Input: part model. Units: mm. Frame: model coordinates. A direction names the side the tool comes from. Give positions to 0.01 mm unless a question says otherwise; leave off trailing zeros. Use CSV: the item, a comma, the result in double quotes.
```python
from build123d import *

# Parameters (mm, degrees)
F0_R     = 3.1
F0_R_2   = 1.75
F1_DEPTH = 16.8
F3_DEPTH = 4
F4_R     = 4
F5_DEPTH = 25
F6_R     = 3


with BuildPart() as f1:
    # F0 (on Top) → F1 (new body)
    with BuildSketch(Plane.XY):
        with BuildLine():
            Line((239.499999, 57.5), (294.438024, 57.5))
            ThreePointArc((294.438024, 57.5), (212.132034, 212.132034), (57.5, 294.438024))
            Line((57.5, 294.438024), (57.5, 239.499999))
            Line((57.5, 239.499999), (-57.5, 239.499999))
            Line((-57.5, 239.499999), (-57.5, 294.438024))
            ThreePointArc((-57.5, 294.438024), (-212.132034, 212.132034), (-294.438024, 57.5))
            Line((-294.438024, 57.5), (-239.499999, 57.5))
            Line((-239.499999, 57.5), (-239.499999, -57.5))
            Line((-239.499999, -57.5), (-294.438024, -57.5))
            ThreePointArc((-294.438024, -57.5), (-212.132034, -212.132034), (-57.5, -294.438024))
            Line((-57.5, -294.438024), (-57.5, -239.499999))
            Line((-57.5, -239.499999), (57.5, -239.499999))
            Line((57.5, -239.499999), (57.5, -294.438024))
            ThreePointArc((57.5, -294.438024), (212.132034, -212.132034), (294.438024, -57.5))
            Line((294.438024, -57.5), (239.499999, -57.5))
            Line((239.499999, -57.5), (239.499999, 57.5))
        make_face()
        with Locations((-41.7, -229.949999)):
            Circle(F0_R, mode=Mode.SUBTRACT)
        with Locations((-229.949999, -41.7)):
            Circle(F0_R, mode=Mode.SUBTRACT)
        with Locations((-50.2, -94.949999)):
            Circle(F0_R, mode=Mode.SUBTRACT)
        with Locations((-94.949999, -50.2)):
            Circle(F0_R, mode=Mode.SUBTRACT)
        with Locations((-4.47245, -35.938702)):
            Circle(F0_R_2, mode=Mode.SUBTRACT)
        with Locations((-35.938702, -4.47245)):
            Circle(F0_R_2, mode=Mode.SUBTRACT)
        with Locations((41.7, -229.949999)):
            Circle(F0_R, mode=Mode.SUBTRACT)
        with Locations((50.2, -94.949999)):
            Circle(F0_R, mode=Mode.SUBTRACT)
        Polygon((-15.5, -66), (-15.5, -45), (15.5, -45), (15.5, -66), (6.5, -66), (6.5, -81), (-6.5, -81), (-6.5, -66), align=None, mode=Mode.SUBTRACT)
        with Locations((94.949999, -50.2)):
            Circle(F0_R, mode=Mode.SUBTRACT)
        with Locations((229.949999, -41.7)):
            Circle(F0_R, mode=Mode.SUBTRACT)
        with Locations((-229.949999, 41.7)):
            Circle(F0_R, mode=Mode.SUBTRACT)
        with Locations((-94.949999, 50.2)):
            Circle(F0_R, mode=Mode.SUBTRACT)
        Polygon((-45, 15.5), (-45, -15.5), (-66, -15.5), (-66, -6.5), (-81, -6.5), (-81, 6.5), (-66, 6.5), (-66, 15.5), align=None, mode=Mode.SUBTRACT)
        with Locations((-50.2, 94.949999)):
            Circle(F0_R, mode=Mode.SUBTRACT)
        with Locations((-41.7, 229.949999)):
            Circle(F0_R, mode=Mode.SUBTRACT)
        with Locations((35.938702, 4.47245)):
            Circle(F0_R_2, mode=Mode.SUBTRACT)
        with Locations((4.47245, 35.938702)):
            Circle(F0_R_2, mode=Mode.SUBTRACT)
        Polygon((66, -15.5), (45, -15.5), (45, 15.5), (66, 15.5), (66, 6.5), (81, 6.5), (81, -6.5), (66, -6.5), align=None, mode=Mode.SUBTRACT)
        Polygon((15.5, 66), (15.5, 45), (-15.5, 45), (-15.5, 66), (-6.5, 66), (-6.5, 81), (6.5, 81), (6.5, 66), align=None, mode=Mode.SUBTRACT)
        with Locations((94.949999, 50.2)):
            Circle(F0_R, mode=Mode.SUBTRACT)
        with Locations((50.2, 94.949999)):
            Circle(F0_R, mode=Mode.SUBTRACT)
        with Locations((229.949999, 41.7)):
            Circle(F0_R, mode=Mode.SUBTRACT)
        with Locations((41.7, 229.949999)):
            Circle(F0_R, mode=Mode.SUBTRACT)
    extrude(amount=F1_DEPTH)

    # F2 (on face) → F3 (cut)
    with BuildSketch(Plane.XY.offset(16.8)):
        Polygon((-144.86168, -16.168246), (-263.65562, -134.962185), (-134.962185, -263.65562), (-16.168246, -144.86168), align=None)
        Polygon((144.86168, -16.168246), (16.168246, -144.86168), (134.962185, -263.65562), (263.65562, -134.962185), align=None)
        Polygon((16.168246, 144.86168), (144.86168, 16.168246), (263.65562, 134.962185), (134.962185, 263.65562), align=None)
        Polygon((-144.86168, 16.168246), (-16.168246, 144.86168), (-134.962185, 263.65562), (-263.65562, 134.962185), align=None)
    extrude(amount=-F3_DEPTH, mode=Mode.SUBTRACT)

    # F4 (on face) → F5 (cut)
    with BuildSketch(Plane.XY.offset(16.8)):
        with Locations((-263.65562, -99.606846)):
            Circle(F4_R)
        with Locations((-99.606846, -263.65562)):
            Circle(F4_R)
        with Locations((99.606846, -263.65562)):
            Circle(F4_R)
        with Locations((263.65562, -99.606846)):
            Circle(F4_R)
        with Locations((263.65562, 99.606846)):
            Circle(F4_R)
        with Locations((99.606846, 263.65562)):
            Circle(F4_R)
        with Locations((-99.606846, 263.65562)):
            Circle(F4_R)
        with Locations((-263.65562, 99.606846)):
            Circle(F4_R)
    extrude(amount=-F5_DEPTH, mode=Mode.SUBTRACT)

    # F6
    f6_edges = [f1.edges().sort_by_distance(p)[0] for p in [
        (57.5, -239.499999, 8.4),
        (57.5, -294.438024, 8.4),
        (-57.5, -239.499999, 8.4),
        (-57.5, -294.438024, 8.4),
        (-294.438024, 57.5, 8.4),
        (-239.499999, 57.5, 8.4),
        (-239.499999, -57.5, 8.4),
        (-294.438024, -57.5, 8.4),
        (57.5, 239.499999, 8.4),
        (294.438024, -57.5, 8.4),
        (57.5, 294.438024, 8.4),
        (-57.5, 239.499999, 8.4),
        (-57.5, 294.438024, 8.4),
        (239.499999, -57.5, 8.4),
        (239.499999, 57.5, 8.4),
        (294.438024, 57.5, 8.4),
    ]]
    fillet(f6_edges, radius=F6_R)


solid = f1.part
```
1) Reachability of faces 3 (the flat face through (81, 0, 8)), 4 (the flat face through (57.5, 267, 8)), 5 (the flat face through (-205.09, 76.397, 14.828)) from +Z, -Z, +X, -X, +Y, -Y: full face, straight path, thin tool, end or side. Return the list, or none.
From the geometry:
face 3,"+Z, -Z"
face 4,"+Z, -Z, +Y"
face 5,"+Z"
2) Contact query for flat-ended pins moving along their axis: pin 1 (1 mm diameter, centred on y = -142, z = 4.5, fed in from +X); pin 2 (13 mm diameter, centred on x = -263.66, y = 99.61, fed in from +Z); pin 3 (6 mm diameter, centred on x = 179, y = 189, fed in from +Z); pin 4 (10 mm diameter, centred on x = 121.5, z = 10.5, fed in from +Y). Output: stop coordinate, or through.
From the geometry:
pin 1,"stops at x = 264.53"
pin 2,"stops at z = 16.8"
pin 3,"stops at z = 12.8"
pin 4,"stops at y = 276.46"
3) Mould query, pull axis X, two halves, no side actions, for faces 1 (the flat face through (-15.5, -56, 8)), 2 (the flat face through (138, 142, 12.8)). Classes: pulls with the +X half, pulls with the -X half, needs draft (parallel to the pull), parting line crosses it, or undercut.
From the geometry:
face 1,"undercut"
face 2,"undercut"
4) Section query A-A (z = 6.25). Give the number of separate pieces and of enclosed holes in the cut face, then the cut area to 3 significant figures.
From the geometry:
separate pieces,"1"
enclosed holes,"32"
area,"251,000 mm^2"
5) Ray query, line 1 (X direction, y = 5, z = 9.75); line 2 (Y direction, x = -8, z = 2.75); line 3 (Y direction, x = -2, z = 5.5). Return the intervals inside material, ascending.
From the geometry:
line 1,"x = -239.5 to -81, -45 to 34.27, 37.61 to 45, 81 to 239.5"
line 2,"y = -239.5 to -66, -45 to 45, 66 to 239.5"
line 3,"y = -239.5 to -81, -45 to 45, 81 to 239.5"
